Can you work these out from the model? Positions are in its coordinate system, mm. Face numbers are marked on the shaded views. Round coordinates to 2 decimals unless told otherwise and drop trailing zeros. Write each loop counter-clockwise with the first axis right and the second up, starting at its lowest first coordinate (ties: lowest second). Pieces come first, ordered by that corner, then holes. Notation, with made-up numbers: (1, -30) - (49, -30) arc R28 cw to (49, 7) - close; hole circle Ø9 at (46.5, 26). An arc over 180 degrees is marked (long way). One line per item, written item: value. Start each with the question number.
(1) I'm going to push flat-ended pins straight in: pin 1 Ø1 at (x, y) = (19, 4) entering from +Z; pin 2 Ø11.5 at (x, z) = (-47.7, 0) entering from -Y; pin 3 Ø1.6 at (y, z) = (15, -10) entering from -X; pin 4 Ø6 at (x, z) = (47.7, 0) entering from +Y. Where does each tip first touch, or does it pass through?
(2) I want a section at A-A on z = 0. List the corners of the cut face in (x, y) for me.
(3) Thinking about a two-plate mould opening in Y: for the marked faces 1, 2, 3 and 4, which applies, +Y half, -Y half, draft (parallel to the pull), parting line (faces both ways), or undercut?
(4) I want a section at B-B on x = -40.5. List the corners of the cut face in (y, z) for me.
(5) I want a section at D-D on y = 8.25. List the corners of the cut face in (x, z) for me.
(6) If I drill on L1, parallel to X at y = 20.8, z = 0; L2, parallel to Y at x = -33.5, z = -5.25; L3, parallel to X at y = 1.5, z = 4.5, over which ranges is the centre line in solid material (lowest first)? Write a range as from..to.
(7) I want a section at C-C on x = 23. List the corners of the cut face in (y, z) for me, plus the area to 3 significant figures.
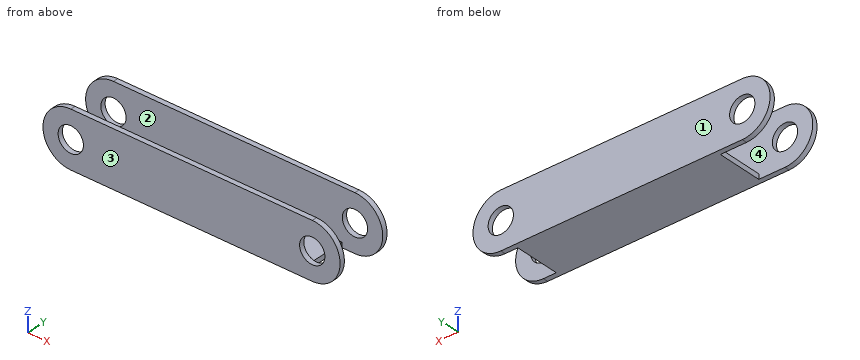
from build123d import *

# Parameters (mm, degrees)
SKETCH1_R           = 5
BOSS_EXTRUDE1_DEPTH = 2
SKETCH2_W           = 80
SKETCH2_H           = 2
BOSS_EXTRUDE2_DEPTH = 9


with BuildPart() as part:
    # Sketch1 → Boss-Extrude1 (new body)
    with BuildSketch(Plane(origin=(0, 0, 0), x_dir=(1, 0, 0), z_dir=(0, 1, 0))):
        with BuildLine():
            Line((-47.7, 11), (47.7, 11))
            ThreePointArc((47.7, 11), (58.7, 0), (47.7, -11))
            Line((47.7, -11), (-47.7, -11))
            ThreePointArc((-47.7, -11), (-58.7, 0), (-47.7, 11))
        make_face()
        with Locations(Location((47.7, 0, 0), (0, 0, 270))):
            Circle(SKETCH1_R, mode=Mode.SUBTRACT)
        with Locations(Location((-47.7, 0, 0), (0, 0, 270))):
            Circle(SKETCH1_R, mode=Mode.SUBTRACT)
    extrude(amount=BOSS_EXTRUDE1_DEPTH)

    # Sketch2 → Boss-Extrude2 (add)
    with BuildSketch(Plane(origin=(0, 2, 0), x_dir=(1, 0, 0), z_dir=(0, 1, 0))):
        with Locations((2.64092049, 10)):
            Rectangle(SKETCH2_W, SKETCH2_H)
    extrude(amount=BOSS_EXTRUDE2_DEPTH)

    # Mirror1: part across plane


with BuildPart() as part_1:
    add(part.part)
    add(part.part.mirror(Plane.ZX.offset(11)))


solid = part_1.part
Established:
1. pin 1: z = -9
1. pin 2: y = 0
1. pin 3: x = -37.36
1. pin 4: through
2. outline: (-58.7, 0) - (-52.7, 0) - (-52.7, 2) - (-58.7, 2) - close; (-58.7, 20) - (-52.7, 20) - (-52.7, 22) - (-58.7, 22) - close; (-42.7, 0) - (42.7, 0) - (42.7, 2) - (-42.7, 2) - close; (-42.7, 20) - (42.7, 20) - (42.7, 22) - (-42.7, 22) - close; (52.7, 0) - (58.7, 0) - (58.7, 2) - (52.7, 2) - close; (52.7, 20) - (58.7, 20) - (58.7, 22) - (52.7, 22) - close
3. face 1: +Y half
3. face 2: undercut
3. face 3: -Y half
3. face 4: undercut
4. outline: (0, -11) - (2, -11) - (2, 11) - (0, 11) - close; (20, -11) - (22, -11) - (22, 11) - (20, 11) - close
5. outline: (-37.36, -11) - (42.64, -11) - (42.64, -9) - (-37.36, -9) - close
6. L1: -58.7..-52.7, -42.7..42.7, 52.7..58.7
6. L2: 0..2, 20..22
6. L3: -57.74..-49.88, -45.52..45.52, 49.88..57.74
7. outline: (0, -11) - (22, -11) - (22, 11) - (20, 11) - (20, -9) - (2, -9) - (2, 11) - (0, 11) - close
7. area: 124 mm2
